The listing builds one solid part. Answer for the finished solid, in the listing's coordinates (mm). A direction names the side the tool comes from. Give positions to 0.01 mm unless a question says otherwise; leave off trailing zeros. Loops run counter-clockwise (first coordinate to the right, second up) from the corner with the lowest first, then second, coordinate; pieces in that order, holes last. Notation, with made-up numbers: M 33.5,36.25 L 52.5,36.25 A20 ccw 52.5,41.25 Z; hole C 78,29 d8. An arc over 180 degrees is marked long. One line per item, written item: value. Start each with the question number.
Q1. A cutting plane is placed at A-A, the plane z = 5.5. Determine the outline of the cut face in (x, y) (3 decimals), and give its area (3 significant figures).
Q2. Flat-ended cylindrical pins translate along their axes: pin 1 (1 mm diameter, centred on y = -10, z = 49, fed in from +X); pin 2 (15.5 mm diameter, centred on x = 0.5, z = 36, fed in from +Y); pin 3 (5 mm diameter, centred on x = 59.5, z = 42, fed in from +Y). Find the tip coordinate at first contact, or state that the pin passes through.
Q3. The mould has two halves that part along X. Classify faces 4 (the cylindrical face through (45.8, -0.4, 38.1)), 5 (the cylindrical face through (32.73, 16.55, 51.97)), 6 (the flat face through (6, 7.938, 30)): +X half, -X half, draft (parallel to the pull), parting line (faces both ways), or undercut.
Q4. A cutting plane is placed at D-D, the plane y = 22. Determine the outline of the cut face in (x, z) (3 decimals), and give its area (3 significant figures).
Q5. For faces 1 (the flat face through (82, 0, 38.1)), 2 (the flat face through (22.225, 17, 18)), 3 (the cylindrical face through (32.73, -16.79, 51.97)), determine the directions among +Z, -Z, +X, -X, +Y, -Y from which every point of the face is accessible in a straight line to the end or side of a thin tool.
Q6. A cutting plane is placed at C-C, the plane x = 78. Determine the outline of the cut face in (y, z) (3 decimals), and give its area (3 significant figures).
Q7. A cutting plane is placed at B-B, the plane y = -19.5. Determine the outline of the cut face in (x, z) (3 decimals).
Q8. Consider L1, parallel to Y at x = 29.5, z = 11.5; L2, parallel to Y at x = 17, z = 27.5; L3, parallel to Z at x = 74, y = -21 (3 decimals). Determine where each line is inside the solid, lowest interval first.
from build123d import *

# Parameters (mm, degrees)
F1_W     = 82.55
F1_H     = 19.05
F2_DEPTH = 63.5
F0_W     = 21.1554604056
F0_H     = 19.05
F3_DEPTH = 25.4
F4_DEPTH = 7.9375
F6_R     = 6.35
F7_R     = 6.35


with BuildPart() as f2:
    # F1 (on Front) → F2 (new body, symmetric)
    with BuildSketch(Plane.XZ):
        Rectangle(F1_W, F1_H)
    extrude(amount=F2_DEPTH, both=True)

    # F0 (on Front) → F3 (join, symmetric)
    with BuildSketch(Plane.XZ):
        with BuildLine():
            Line((22.225, 9.525), (41.275, 9.525))
            Line((41.275, 9.525), (41.275, 27.0002))
            ThreePointArc((41.275, 27.0002), (45.9246798487, 38.2255201513), (57.15, 42.8752))
            Line((57.15, 42.8752), (60.325, 42.8752))
            Line((60.325, 42.8752), (60.325, 61.9252))
            Line((60.325, 61.9252), (57.15, 61.9252))
            ThreePointArc((57.15, 61.9252), (32.4542956671, 51.6959043329), (22.225, 27.0002))
            Line((22.225, 27.0002), (22.225, 9.525))
        make_face()
        with Locations((70.9027302028, 52.4002)):
            Rectangle(F0_W, F0_H)
    extrude(amount=F3_DEPTH, both=True)

    # F0 (on Front) → F4 (join, symmetric)
    with BuildSketch(Plane.XZ):
        with BuildLine():
            add(Edge.make_bspline(
                [(-41.275, 9.525), (-27.3804180324, 35.7423387468), (15.3577309102, 62.309294939), (57.15, 61.9252)],
                knots=[0, 0, 0, 0, 111.5045361635, 111.5045361635, 111.5045361635, 111.5045361635], degree=3))
            Line((-41.275, 9.525), (22.225, 9.525))
            Line((22.225, 9.525), (22.225, 27.0002))
            ThreePointArc((22.225, 27.0002), (32.4542956671, 51.6959043329), (57.15, 61.9252))
        make_face()
    extrude(amount=F4_DEPTH, both=True)

    # F0 (on Front) → F5 (revolve)
    with BuildSketch(Plane.XZ):
        Polygon((81.4804604056, 66.675), (81.4804604056, 61.9252), (81.4804604056, 42.8752), (81.4804604056, 38.1), (111.125, 38.1), (111.125, 66.675), align=None)
    revolve(axis=Axis((81.4804604056, 0, 52.3875), (0, 0, 1)))

    # F6
    f6_edges = [f2.edges().sort_by_distance(p)[0] for p in [
        (41.275, -63.5, 0),
        (-41.275, -63.5, 0),
        (41.275, 63.5, 0),
    ]]
    fillet(f6_edges, radius=F6_R)

    # F7
    f7_edges = [f2.edges().sort_by_distance(p)[0] for p in [
        (-41.275, 63.5, 0),
    ]]
    fillet(f7_edges, radius=F7_R)


solid = f2.part
Answer block:
1. outline: M -41.275,-57.15 A6.35 ccw -34.925,-63.5 L 34.925,-63.5 A6.35 ccw 41.275,-57.15 L 41.275,57.15 A6.35 ccw 34.925,63.5 L -34.925,63.5 A6.35 ccw -41.275,57.15 Z
1. area: 10,400 mm^2
2. pin 1: x = 109.56
2. pin 2: y = 7.94
2. pin 3: y = 25.4
3. face 4: undercut
3. face 5: -X half
3. face 6: draft
4. outline: M -41.275,-9.525 L 41.275,-9.525 L 41.275,27 A15.875 cw 57.15,42.875 L 61.611,42.875 L 61.611,38.1 L 101.35,38.1 L 101.35,66.675 L 61.611,66.675 L 61.611,61.925 L 57.15,61.925 A34.925 ccw 22.225,27 L 22.225,9.525 L -41.275,9.525 Z
4. area: 3,890 mm^2
5. face 1: -Z, +X, +Y, -Y
5. face 2: +Z, -X, +Y
5. face 3: +Z, -X, -Y
6. outline: M -29.44,38.1 L 29.44,38.1 L 29.44,66.675 L -29.44,66.675 Z
6. area: 1,680 mm^2
7. outline: M -41.275,-9.525 L 41.275,-9.525 L 41.275,27 A15.875 cw 57.15,42.875 L 59.152,42.875 L 59.152,38.1 L 103.809,38.1 L 103.809,66.675 L 59.152,66.675 L 59.152,61.925 L 57.15,61.925 A34.925 ccw 22.225,27 L 22.225,9.525 L -41.275,9.525 Z
8. L1: -25.4 to 25.4
8. L2: -7.94 to 7.94
8. L3: 38.1 to 66.675
